from build123d import *

# Parameters (mm, degrees)
F1_DEPTH = 19.05
F3_D     = 15.0114
F3_DEPTH = 14.224
F3_TIP   = 4.5098795482
F5_D     = 8.001
F5_DEPTH = 25.4
F5_TIP   = 2.4037429064
F7_D     = 8.001
F7_DEPTH = 25.4
F7_TIP   = 2.4037429064


# Not quite as in the source:
# - a feature names something its author has since deleted; it is built from what else it names


with BuildPart() as f1:
    # F0 (on Top) → F1 (new body)
    with BuildSketch(Plane.XY):
        Polygon((285.75, -295.275), (285.75, 295.275), (0, 295.275), (-285.75, 295.275), (-285.75, -295.275), align=None)
        with BuildLine():
            ThreePointArc((30.1625, 219.075), (-21.3281082875, 197.7468917125), (0, 249.2375))
            ThreePointArc((0, 249.2375), (21.3281082875, 240.4031082875), (30.1625, 219.075))
        make_face(mode=Mode.SUBTRACT)
    extrude(amount=F1_DEPTH)

    # F3
    with Locations(Plane(origin=(0, 0, 0), x_dir=(1, 0, 0), z_dir=(0, 0, -1))):
        with Locations((-261.874, 244.475), (261.874, 244.475), (-261.874, 0), (261.874, 0), (261.874, -244.475), (-261.874, -244.475)):
            Hole(F3_D / 2, depth=F3_DEPTH)
            with Locations((0, 0, -(F3_DEPTH + F3_TIP / 2))):  # 118° drill point
                Cone(0, F3_D / 2, F3_TIP, mode=Mode.SUBTRACT)

    # F5
    with Locations(Plane.YZ.offset(285.75)):
        with Locations((-244.475, 9.525), (0, 9.525), (233.3625, 9.525)):
            Hole(F5_D / 2, depth=F5_DEPTH)
            with Locations((0, 0, -(F5_DEPTH + F5_TIP / 2))):  # 118° drill point
                Cone(0, F5_D / 2, F5_TIP, mode=Mode.SUBTRACT)

    # F7
    with Locations(Plane(origin=(-285.75, 0, 0), x_dir=(0, -1, 0), z_dir=(-1, 0, 0))):
        with Locations((0, 9.525), (244.475, 9.525), (-244.475, 9.525)):
            Hole(F7_D / 2, depth=F7_DEPTH)
            with Locations((0, 0, -(F7_DEPTH + F7_TIP / 2))):  # 118° drill point
                Cone(0, F7_D / 2, F7_TIP, mode=Mode.SUBTRACT)


solid = f1.part
Work out the finished part from the listing and answer in its coordinate system (mm). A direction names the side the tool comes from. Give positions to 0.01 mm unless a question says otherwise; leave off trailing zeros. Use a Markdown table: item, result. Add a question column.
1) Consider line 1 along Z through (x, y) = (281, 0); line 2 along X through (y, z) = (203, 2.75); line 3 along Y through (x, z) = (-4, 3.75) (3 decimals). Determine where each line is inside the solid, lowest interval first.
2) Each of these flat-tipped pins is pushed along its axis until it touches: P1, Ø7, axis at y = 0, z = 9.525, coming from the -X side; P2, Ø9, axis at x = -261.874, y = -244.475, coming from the -Z side; P3, Ø7, axis at y = -244.475, z = 9.525, coming from the +X side. Where does it stop, or does it pass through?
3) Which of the six approach directions +Z, -Z, +X, -X, +Y, -Y give full straight-line access (tool end or side, diameter ignored) to faces 4 (the cylindrical face through (254.715, -246.73, 7.212)), 5 (the flat face through (-4, -295.275, 9))?
4) For a pull along X with two mould halves and no side action, classify faces 1 (the conical face through (-261.17, -245.57, 17.95)), 2 (the flat face through (-285.75, 4, 12)), 3 (the flat face through (285.75, -4, 12)) as +X half, -X half, draft (parallel to the pull), parting line (faces both ways), or undercut.
Reported:
| question | item | result |
|---|---|---|
| 1 | line 1 | z = 0 to 5.52, 13.53 to 19.05 |
| 1 | line 2 | x = -285.75 to -25.52, 25.52 to 285.75 |
| 1 | line 3 | y = -295.275 to 189.179, 248.971 to 295.275 |
| 2 | P1 | stops at x = -255.23 |
| 2 | P2 | stops at z = 16.03 |
| 2 | P3 | stops at x = 255.23 |
| 3 | face 4 | -Z |
| 3 | face 5 | +Z, -Z, +X, -X, -Y |
| 4 | face 1 | undercut |
| 4 | face 2 | -X half |
| 4 | face 3 | +X half |
